Check sheet for the modelled part. Datum: model origin and axes. Units: mm. A direction names the side the tool comes from. Give positions to 0.01 mm unless a question says otherwise; leave off trailing zeros. Order: outer loops, then holes, each group sorted by start corner. A loop starts at its lowest first (then second) coordinate and runs counter-clockwise, first axis right, second up.
```python
from build123d import *

# Parameters (mm, degrees)
PAD_DEPTH       = 8
SKETCH001_R     = 2
POCKET_DEPTH    = 5
SKETCH002_R     = 2
POCKET001_DEPTH = 5


with BuildPart() as part:
    # Sketch → Pad (new body)
    with BuildSketch(Plane.XZ):
        Polygon((4, 4), (4, 25), (0, 25), (0, 0), (25, 0), (25, 4), align=None)
    extrude(amount=PAD_DEPTH)

    # Sketch001 (on Face6 of Pad) → Pocket (cut)
    with BuildSketch(Plane(origin=(0, 0, 4), x_dir=(-1, 0, 0), z_dir=(0, 0, 1))):
        with Locations((-20, 4)):
            Circle(SKETCH001_R)
    extrude(amount=-POCKET_DEPTH, mode=Mode.SUBTRACT)

    # Sketch002 (on Face1 of Pocket) → Pocket001 (cut)
    with BuildSketch(Plane(origin=(4, 0, 0), x_dir=(0, 0, 1), z_dir=(1, 0, 0))):
        with Locations((20, 4)):
            Circle(SKETCH002_R)
    extrude(amount=-POCKET001_DEPTH, mode=Mode.SUBTRACT)


solid = part.part
```
(1) Set-up check for faces 5 (the face through (4, -4, 14)), 6 (the face through (12, -4, 0)): record each of +Z, -Z, +X, -X, +Y, -Y from which the full face is reachable in a straight line by a thin tool's end or side.
Response values:
face 5: +Z, +X, +Y, -Y
face 6: -Z, +X, -X, +Y, -Y
(2) Cross-section at D-D on y = -6.5. Enter the section's corners in (x, z), then the cut area to 3 significant figures.
Response values:
outline: (0, 0) - (25, 0) - (25, 4) - (4, 4) - (4, 25) - (0, 25) - close
area: 184 mm2
(3) Cross-section at B-B on y = -3. Enter the section's corners in (x, z), then the cut area to 3 significant figures.
Response values:
outline: (0, 0) - (18.27, 0) - (18.27, 4) - (4, 4) - (4, 18.27) - (0, 18.27) - close; (0, 21.73) - (4, 21.73) - (4, 25) - (0, 25) - close; (21.73, 0) - (25, 0) - (25, 4) - (21.73, 4) - close
area: 156 mm2
(4) Gauge pin test, flat ends, axial feed: pin 1 Ø1.5 at (x, y) = (22.5, -3.5) entering from +Z; pin 2 Ø4 at (x, y) = (4.5, -6) entering from -Z; pin 3 Ø12 at (x, z) = (12, 16.5) entering from +Y (3 decimals); pin 4 Ø4 at (y, z) = (-4.5, 18.5) entering from +X. Record the tip position at first contact, or that the pin passes through.
Response values:
pin 1: stops at z = 4
pin 2: stops at z = 0
pin 3: passes through
pin 4: stops at x = 4
(5) Cross-section at C-C on x = 20. Enter the section's corners in (y, z).
Response values:
outline: (-8, 0) - (-6, 0) - (-6, 4) - (-8, 4) - close; (-2, 0) - (0, 0) - (0, 4) - (-2, 4) - close
(6) Cross-section at A-A on z = 20. Enter the section's corners in (x, y), then the cut area to 3 significant figures.
Response values:
outline: (0, -8) - (4, -8) - (4, -6) - (0, -6) - close; (0, -2) - (4, -2) - (4, 0) - (0, 0) - close
area: 16.0 mm2
(7) Material ranges on L1, parallel to Z at x = 2.35, y = -4; L2, parallel to Y at x = 20, z = 0.8, recorded low to high.
Response values:
L1: z = 0 to 18, 22 to 25
L2: y = -8 to -6, -2 to 0
(8) Release check for a two-part mould opening along Y. For faces 1 (the face through (3, 0, 8)), 2 (the face through (3, -8, 8)), 3 (the face through (2, -2.8, 18.4)), 4 (the face through (15, -4, 4)) record: released by +Y, released by -Y, zero draft, split by the parting line, or undercut.
Response values:
face 1: released by +Y
face 2: released by -Y
face 3: undercut
face 4: zero draft
